For this review, take the finished solid that the model builds, in its own axes (mm). A direction names the side the tool comes from. Give positions to 0.01 mm unless a question says otherwise; leave off trailing zeros. Loops run counter-clockwise (first coordinate to the right, second up) from the corner with the lowest first, then second, coordinate; pieces in that order, holes last. Notation, with made-up numbers: (66.5, 81) - (122.5, 81) arc R26 ccw to (122.5, 107) - close; hole circle Ø10 at (3.5, 26.5). An arc over 180 degrees is marked (long way). Answer as CSV lines item,"result".
from build123d import *

# Parameters (mm, degrees)
F0_R     = 5
F0_R_2   = 2
F1_DEPTH = 8
F0_R_3   = 7
F2_DEPTH = 1
F3_R     = 7
F3_R_2   = 5
F4_DEPTH = 1


with BuildPart() as f1:
    # F0 (on Top) → F1 (new body)
    with BuildSketch(Plane.XY):
        Circle(F0_R)
        Circle(F0_R_2, mode=Mode.SUBTRACT)
    extrude(amount=F1_DEPTH)

    # F0 (on Top) → F2 (join)
    with BuildSketch(Plane.XY):
        Circle(F0_R_3)
        Circle(F0_R, mode=Mode.SUBTRACT)
    extrude(amount=F2_DEPTH)

    # F3 (on face) → F4 (join)
    with BuildSketch(Plane.XY.offset(8)):
        Circle(F3_R)
        Circle(F3_R_2, mode=Mode.SUBTRACT)
    extrude(amount=-F4_DEPTH)


solid = f1.part
1) Insertion check: P1, Ø1, axis at x = -4.5, z = 3.5, coming from the +Y side; P2, Ø2, axis at y = -4, z = 3.5, coming from the -X side; P3, Ø1.5, axis at x = 3.5, z = 4, coming from the -Y side; P4, Ø4.5, axis at x = 0, y = 0, coming from the -Z side. Each pin has a flat end and moves straight along its axis. Give the tip position at first contact, or say it passes through.
From the geometry:
P1,"stops at y = 3"
P2,"stops at x = -4"
P3,"stops at y = -4.18"
P4,"stops at z = 0"
2) Consider section D-D on y = -4. Write out the cut boundary in (x, z), and give its area (3 significant figures).
From the geometry:
outline,"(-5.74, 0) - (5.74, 0) - (5.74, 1) - (3, 1) - (3, 7) - (5.74, 7) - (5.74, 8) - (-5.74, 8) - (-5.74, 7) - (-3, 7) - (-3, 1) - (-5.74, 1) - close"
area,"59.0 mm^2"
3) Draft analysis for pull direction Z (two halves, no side actions). For faces 1 (the cylindrical face through (0, -2, 4)), 2 (the flat face through (1, 2, 8)), 3 (the flat face through (-2, 5, 1)), state which applies: pulls with the +Z half, pulls with the -Z half, needs draft (parallel to the pull), parting line crosses it, or undercut.
From the geometry:
face 1,"needs draft"
face 2,"pulls with the +Z half"
face 3,"undercut"
4) Consider section A-A on y = 0. Write out the cut boundary in (x, z).
From the geometry:
outline,"(-7, 0) - (-2, 0) - (-2, 8) - (-7, 8) - (-7, 7) - (-5, 7) - (-5, 1) - (-7, 1) - close; (2, 0) - (7, 0) - (7, 1) - (5, 1) - (5, 7) - (7, 7) - (7, 8) - (2, 8) - close"
5) Wall thickness on line 1 (Z direction, x = 6.25, y = 3); line 2 (Y direction, x = 0, z = 4); line 3 (Y direction, x = 1.75, z = 0.5): over which ranges is each line inside the solid? List them lowest first. Write a range as from..to.
From the geometry:
line 1,"z = 0..1, 7..8"
line 2,"y = -5..-2, 2..5"
line 3,"y = -6.78..-0.97, 0.97..6.78"
6) Consider section C-C on z = 3.75. Write out the cut boundary in (x, y), and give its area (3 significant figures).
From the geometry:
outline,"circle Ø10 at (0, 0); hole circle Ø4 at (0, 0)"
area,"66.0 mm^2"
7) Machinability: for faces 4 (the cylindrical face through (-1.08, -4.88, 3.96)), 5 (the cylindrical face through (6.466, -2.681, 0.493)), which of the approach directions +Z, -Z, +X, -X, +Y, -Y give a long, thin tool a straight path to every point of the face, cutting with its end or side? Answer none if there is none.
From the geometry:
face 4,"none"
face 5,"+Z, -Z"
